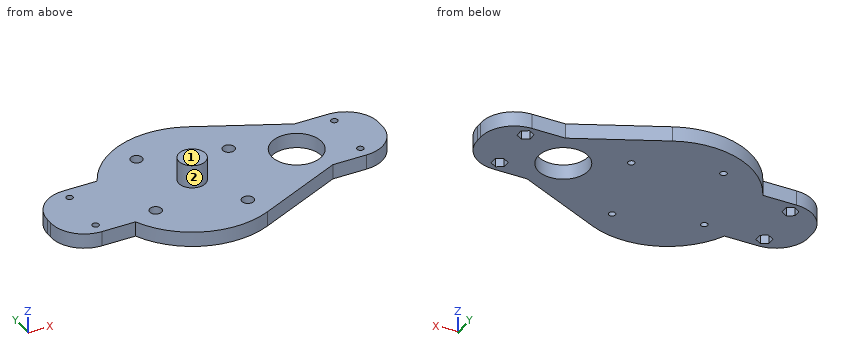
from build123d import *

# Parameters (mm, degrees)
BOSS_EXTRUDE1_DEPTH = 4.5
SKETCH2_R           = 7.5
CUT_EXTRUDE1_DEPTH  = 50.942466899
SKETCH3_R           = 4
BOSS_EXTRUDE2_DEPTH = 7
BOSS_EXTRUDE3_DEPTH = 4.5
FILLET1_R           = 10
SKETCH6_R           = 1
CUT_EXTRUDE2_DEPTH  = 63.42486639
CUT_EXTRUDE3_DEPTH  = 3
SKETCH10_R          = 1
CUT_EXTRUDE4_DEPTH  = 62.754464971
SKETCH11_R          = 1.775
CUT_EXTRUDE5_DEPTH  = 2.5


with BuildPart() as part:
    # Sketch1 → Boss-Extrude1 (new body)
    with BuildSketch(Plane.XY):
        with BuildLine():
            Line((10.483870968, 22.695560128), (36.032258065, 10.893868862))
            ThreePointArc((36.032258065, 10.893868862), (43, 0), (36.032258065, -10.893868862))
            Line((36.032258065, -10.893868862), (10.483870968, -22.695560128))
            ThreePointArc((10.483870968, -22.695560128), (-25, 0), (10.483870968, 22.695560128))
        make_face()
    extrude(amount=BOSS_EXTRUDE1_DEPTH)

    # Sketch2 → Cut-Extrude1 (cut, through all)
    with BuildSketch(Plane.XY.offset(4.5)):
        with Locations((31, 0)):
            Circle(SKETCH2_R)
    extrude(amount=-CUT_EXTRUDE1_DEPTH, mode=Mode.SUBTRACT)

    # Sketch3 → Boss-Extrude2 (add)
    with BuildSketch(Plane.XY.offset(4.5)):
        Circle(SKETCH3_R)
    extrude(amount=BOSS_EXTRUDE2_DEPTH)

    # Sketch4 → Boss-Extrude3 (add)
    with BuildSketch(Plane(origin=(0, 0, 0), x_dir=(-1, 0, 0), z_dir=(0, 0, -1))):
        with BuildLine():
            Line((-36.032258065, 10.893868862), (-56.032258065, 10.893868862))
            Line((-56.032258065, 10.893868862), (-56.032258065, -10.893868862))
            Line((-56.032258065, -10.893868862), (-36.032258065, -10.893868862))
            ThreePointArc((-36.032258065, -10.893868862), (-43, 0), (-36.032258065, 10.893868862))
        make_face()
        with BuildLine():
            Line((22.501635968, 10.893868862), (42.501635968, 10.893868862))
            Line((42.501635968, 10.893868862), (42.501635968, -10.893868862))
            Line((42.501635968, -10.893868862), (22.501635968, -10.893868862))
            ThreePointArc((22.501635968, -10.893868862), (25, 0), (22.501635968, 10.893868862))
        make_face()
    extrude(amount=-BOSS_EXTRUDE3_DEPTH)

    # Fillet1
    fillet1_edges = [part.edges().sort_by_distance(p)[0] for p in [
        (56.032258065, 10.893868862, 2.25),
        (56.032258065, -10.893868862, 2.25),
        (-42.501635968, -10.893868862, 2.25),
        (-42.501635968, 10.893868862, 2.25),
    ]]
    fillet(fillet1_edges, radius=FILLET1_R)

    # Sketch6 → Cut-Extrude2 (cut, through all)
    with BuildSketch(Plane(origin=(0, 0, 0), x_dir=(-1, 0, 0), z_dir=(0, 0, -1))):
        with Locations((32.501635968, -7.384406603)):
            Circle(SKETCH6_R)
        with Locations((32.501635968, 7.384406603)):
            Circle(SKETCH6_R)
        with Locations((-46.032258065, -7.384406603)):
            Circle(SKETCH6_R)
        with Locations((-46.032258065, 7.384406603)):
            Circle(SKETCH6_R)
    extrude(amount=-CUT_EXTRUDE2_DEPTH, mode=Mode.SUBTRACT)

    # Sketch7 → Cut-Extrude3 (cut)
    with BuildSketch(Plane(origin=(0, 0, 0), x_dir=(-1, 0, 0), z_dir=(0, 0, -1))):
        Polygon((-46.040823363, 9.636056412), (-47.986526649, 8.502813742), (-47.97796135, 6.251163933), (-46.023692766, 5.132756795), (-44.07798948, 6.265999465), (-44.086554779, 8.517649274), align=None)
        Polygon((-46.040823363, -5.132756795), (-47.986526649, -6.265999465), (-47.97796135, -8.517649274), (-46.023692766, -9.636056412), (-44.07798948, -8.502813742), (-44.086554779, -6.251163933), align=None)
        Polygon((32.500854226, 9.636072568), (30.551245171, 8.509562577), (30.552026913, 6.257896613), (32.502417709, 5.132740639), (34.452026765, 6.259250629), (34.451245023, 8.510916594), align=None)
        Polygon((32.500854226, -5.132740639), (30.551245171, -6.259250629), (30.552026913, -8.510916594), (32.502417709, -9.636072568), (34.452026765, -8.509562577), (34.451245023, -6.257896613), align=None)
    extrude(amount=-CUT_EXTRUDE3_DEPTH, mode=Mode.SUBTRACT)

    # Sketch10 → Cut-Extrude4 (cut, through all)
    with BuildSketch(Plane.XY.offset(4.5)):
        with Locations((8.530630169, -15.279998329)):
            Circle(SKETCH10_R)
        with Locations((-15.279998329, -8.530630169)):
            Circle(SKETCH10_R)
        with Locations((-8.530630169, 15.279998329)):
            Circle(SKETCH10_R)
        with Locations((15.279998329, 8.530630169)):
            Circle(SKETCH10_R)
    extrude(amount=-CUT_EXTRUDE4_DEPTH, mode=Mode.SUBTRACT)

    # Sketch11 → Cut-Extrude5 (cut)
    with BuildSketch(Plane.XY.offset(4.5)):
        with Locations((-8.530630169, 15.279998329)):
            Circle(SKETCH11_R)
        with Locations((15.279998329, 8.530630169)):
            Circle(SKETCH11_R)
        with Locations((8.530630169, -15.279998329)):
            Circle(SKETCH11_R)
        with Locations((-15.279998329, -8.530630169)):
            Circle(SKETCH11_R)
    extrude(amount=-CUT_EXTRUDE5_DEPTH, mode=Mode.SUBTRACT)


solid = part.part
Could you check a few things on this model? Use its own coordinates, in mm. Face numbers are marked on the shaded views. A direction names the side the tool comes from. Give positions to 0.01 mm unless a question says otherwise; leave off trailing zeros. Order: outer loops, then holes, each group sorted by start corner. A loop starts at its lowest first (then second) coordinate and runs counter-clockwise, first axis right, second up.
Item 1: I'm going to push flat-ended pins straight in: pin 1 (4 mm diameter, centred on x = 15.28, y = 8.53, fed in from +Z); pin 2 (1.1 mm diameter, centred on y = -7.5, z = 1.5, fed in from -X); pin 3 (4 mm diameter, centred on x = -2, z = 1.5, fed in from +Y). Where does each tip first touch, or does it pass through?
Item 2: If we section it at B-B, the plane x = 0: Write out the boundary of the cut face in (y, z).
Item 3: If we section it at D-D, the plane x = 29: Write out the boundary of the cut face in (y, z), plus the area to 3 significant figures.
Item 4: If we section it at A-A, the plane y = 0: Write out the boundary of the cut face in (x, z).
Item 5: If we section it at C-C, the plane z = 6: Write out the boundary of the cut face in (x, y).
Item 6: I need wall thicknesses on line 1 (X direction, y = -3, z = 0.75); line 2 (Z direction, x = 40, y = 1.5); line 3 (Y direction, x = 34, z = 2.25). Which ranges of each line are inside material? Lowest first, please.
Item 7: For the marked faces 1 and 2, which set-ups out of +Z, -Z, +X, -X, +Y, -Y let a thin tool reach every point of the face, with its end or its side?
Values:
1. pin 1: stops at z = 4.5
1. pin 2: stops at x = -40.46
1. pin 3: stops at y = 25
2. outline: (-25, 0) - (25, 0) - (25, 4.5) - (4, 4.5) - (4, 11.5) - (-4, 11.5) - (-4, 4.5) - (-25, 4.5) - close
3. outline: (-14.14, 0) - (-7.23, 0) - (-7.23, 4.5) - (-14.14, 4.5) - close; (7.23, 0) - (14.14, 0) - (14.14, 4.5) - (7.23, 4.5) - close
3. area: 62.2 mm2
4. outline: (-42.5, 0) - (23.5, 0) - (23.5, 4.5) - (4, 4.5) - (4, 11.5) - (-4, 11.5) - (-4, 4.5) - (-42.5, 4.5) - close; (38.5, 0) - (56.03, 0) - (56.03, 4.5) - (38.5, 4.5) - close
5. outline: circle Ø8 at (0, 0)
6. line 1: x = -42.28 to 24.13, 37.87 to 55.81
6. line 2: z = 0 to 4.5
6. line 3: y = -11.83 to -6.87, 6.87 to 11.83
7. face 1: +Z, +X, -X, +Y, -Y
7. face 2: +Z
